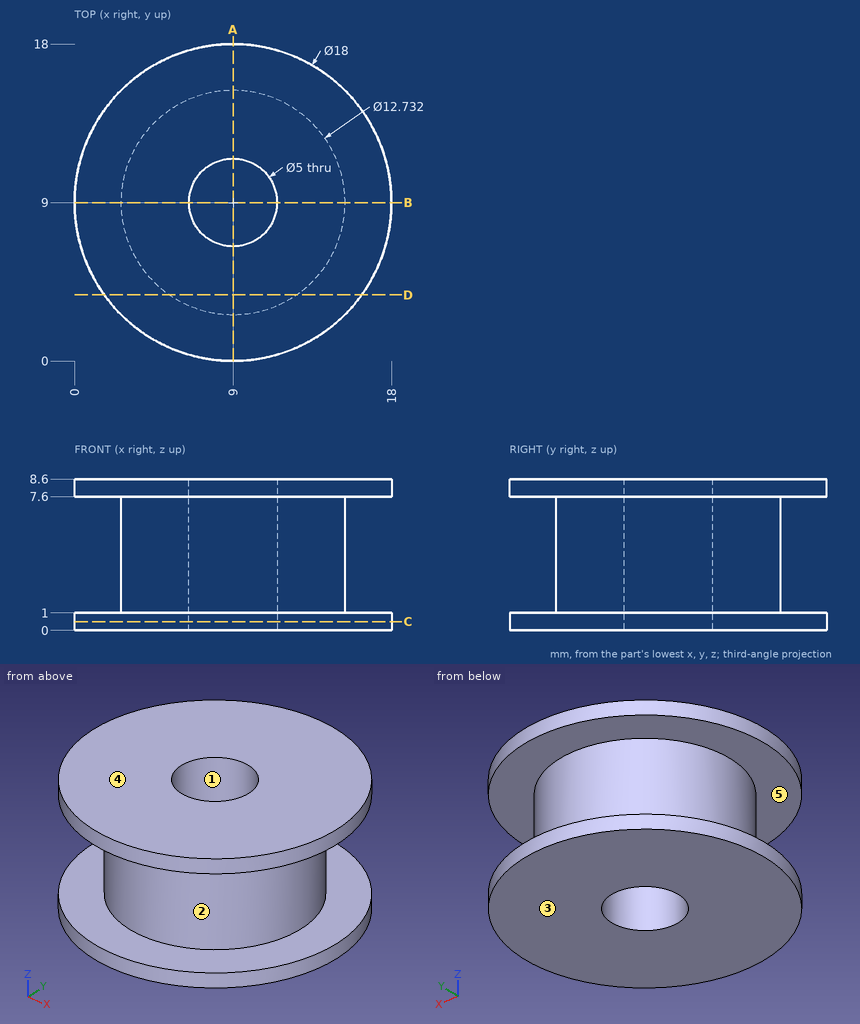
Can you work these out from the drawing? Everything is in mm from the part's minimum corner. A direction names the side the tool comes from. Give positions to 0.01 mm unless a question says otherwise; leave off trailing zeros. Order: outer loops, then holes, each group sorted by start corner. A loop starts at its lowest first (then second) coordinate and runs counter-clockwise, first axis right, second up. Notation, with made-up numbers: (30, -36.75) -> (88, -36.75) arc R21 cw to (88, -23.75) -> close; hole circle Ø3 at (52, 16.5). An arc over 180 degrees is marked (long way). Return JSON: item names as keys, results as strings.
1. Imagine slicing it at D-D on y = 3.75. List the corners of the cut face in (x, z) for me.
Answer list:
{"outline": "(1.69, 0) -> (16.31, 0) -> (16.31, 1) -> (12.6, 1) -> (12.6, 7.6) -> (16.31, 7.6) -> (16.31, 8.6) -> (1.69, 8.6) -> (1.69, 7.6) -> (5.4, 7.6) -> (5.4, 1) -> (1.69, 1) -> close"}
2. Imagine slicing it at C-C on z = 0.5. List the corners of the cut face in (x, y) for me, then the cut area to 3 significant figures.
Answer list:
{"outline": "circle Ø18 at (9, 9); hole circle Ø5 at (9, 9)", "area": "235 mm2"}
3. I need wall thicknesses on line 1 (Z direction, x = 3.25, y = 15.75); line 2 (Y direction, x = 9, z = 4); line 3 (X direction, y = 8.25, z = 4) (1 decimal). Which ranges of each line are inside material? Lowest first, please. Write a range as from..to.
Answer list:
{"line 1": "z = 0..1, 7.6..8.6", "line 2": "y = 2.63..6.5, 11.5..15.37", "line 3": "x = 2.7..6.6, 11.4..15.3"}
4. Thinking about a two-plate mould opening in Y: for the marked faces 1, 2 and 3, which applies, pulls with the +Y half, pulls with the -Y half, needs draft (parallel to the pull), parting line crosses it, or undercut?
Answer list:
{"face 1": "undercut", "face 2": "parting line crosses it", "face 3": "needs draft"}
5. For pin 1 Ø6 at (x, y) = (9.5, 4) entering from -Z; pin 2 Ø5 at (y, z) = (6.5, 6.5) entering from -X; pin 3 Ø1.5 at (y, z) = (12.5, 2) entering from -X, each with a flat end and sliding along its axis, tell me the tip position at first contact or that it passes through.
Answer list:
{"pin 1": "stops at z = 0", "pin 2": "stops at x = 0", "pin 3": "stops at x = 3.26"}
6. On a 3-axis mill with a long thin cutter (end or side, diameter ignored), from which of +Z, -Z, +X, -X, +Y, -Y can I reach the whole of each face in a straight line? I mean the marked faces 4 and 5. Say none if no direction works.
Answer list:
{"face 4": "+Z, +X, -X, +Y, -Y", "face 5": "none"}
7. Imagine slicing it at A-A on x = 9. List the corners of the cut face in (y, z) for me.
Answer list:
{"outline": "(0, 0) -> (6.5, 0) -> (6.5, 8.6) -> (0, 8.6) -> (0, 7.6) -> (2.63, 7.6) -> (2.63, 1) -> (0, 1) -> close; (11.5, 0) -> (18, 0) -> (18, 1) -> (15.37, 1) -> (15.37, 7.6) -> (18, 7.6) -> (18, 8.6) -> (11.5, 8.6) -> close"}
